Autodesk Inventor part; units mm, degrees
ref_plane "YZ Plane" through (0, 0, 0) normal (1, 0, 0) x (0, 1, 0)
ref_plane "XZ Plane" through (0, 0, 0) normal (0, 1, 0) x (-1, 0, 0)
ref_plane "XY Plane" through (0, 0, 0) normal (0, 0, 1) x (1, 0, 0)
sketch "Szkic1" plane through (0, 0, 0) normal (0, 0, 1) x (1, 0, 0)
  circle A0 centre (0, 0) radius 30
  circle A1 centre (0, 0) radius 34
  dimension "d0" = 60
  dimension "d1" = 4
extrude "Wyciągnięcie proste1" add sketch "Szkic1" along normal blind 65
sketch "Szkic2" plane through (0, 0, 65) normal (0, 0, 1) x (1, 0, 0)
  circle A0 centre (35, 0) radius 5
  circle A1 centre (0, 0) radius 34
  circle A2 centre (0, 0) radius 30
  circle A3 centre (35, 0) radius 1.5
  line L0 (0, 0) -> (0, -30)
  circle A4 centre (-35, 0) radius 5
  circle A5 centre (-35, 0) radius 1.5
  point P0 (33.9821, 1.1018)
  point P1 (33.9821, -1.1018)
  point P2 (33.6571, -4.8163)
  point P3 (33.6571, 4.8163)
  point P4 (-33.9821, -1.1018)
  point P5 (-33.9821, 1.1018)
  point P6 (-33.6571, 4.8163)
  point P7 (-33.6571, -4.8163)
  dimension "d5" = 10
  dimension "d6" = 3
  dimension "d9" = 70
extrude "Wyciągnięcie proste2" add sketch "Szkic2" against normal blind 10 contours A0 A1 A3 | A1 A5 A4 picked at (35.0063, -3.323) picked at (-35.0802, 3.3077)
sketch "Szkic3" plane through (0, 0, 65) normal (0, 0, 1) x (1, 0, 0)
  point P0 (0, 0)
sketch "Szkic4" plane through (0, 0, 65) normal (0, 0, 1) x (1, 0, 0)
  arc A0 (-33.9821, 1.1018) -> (-33.9821, -1.1018) centre (-35, 0) ccw
  circle A1 centre (-35, 0) radius 1.5
  arc A2 (33.9821, -1.1018) -> (33.9821, 1.1018) centre (35, 0) ccw
  circle A3 centre (35, 0) radius 1.5
  point P0 (0, 0)
  point P1 (33.9821, 1.1018)
  point P2 (33.9821, -1.1018)
  point P3 (-33.9821, -1.1018)
  point P4 (-33.9821, 1.1018)
extrude "Wyciągnięcie proste3" cut sketch "Szkic4" against normal blind 10
properties part number "osłonasilnik" material "Tworzywo sztuczne PET"
Can you work these out from the model? Positions are in its coordinate system, mm. A direction names the side the tool comes from. Coordinates: 2 decimals unless noted, no trailing zeros. Write each loop counter-clockwise with the first axis right and the second up, starting at its lowest first coordinate (ties: lowest second). Pieces come first, ordered by that corner, then holes. Notation, with made-up numbers: (-27.75, -17) - (30.25, -17) arc R21 cw to (30.25, 19) - close; hole circle Ø1 at (23.25, 26.5). An arc over 180 degrees is marked (long way). Return JSON: item names as keys, results as strings. Group by question number.
Item 1: If we section it at D-D (z = 56): Write out the boundary of the cut face in (x, y).
Item 2: I'm going to push flat-ended pins straight in: pin 1 Ø1.5 at (y, z) = (12.5, 7) entering from +X; pin 2 Ø5 at (x, z) = (29.5, 25) entering from -Y; pin 3 Ø8 at (x, z) = (22, 16.5) entering from -Y. Where does each tip first touch, or does it pass through?
Item 3: We'd pull the mould along Y, two halves only. Please class faces 3 (the face through (32.43, -10.21, 32.04)), 4 (the face through (-37, 0, 55)), 5 (the face through (36.5, 0, 60.1)): pulls with the +Y half, pulls with the -Y half, needs draft (parallel to the pull), parting line crosses it, or undercut.
Item 4: Please list where these lines run through material, in increasing order: probe 1 along Y at (x, z) = (0, 39.5); probe 2 along X at (y, z) = (1, 30.5); probe 3 along Y at (x, z) = (-35, 63).
Item 5: If we section it at B-B (y = 0): Write out the boundary of the cut face in (x, z), then the cut area to 3 significant figures.
Item 6: Which directions (+Z, -Z, +X, -X, +Y, -Y) give clear straight access to the entire face, cutting with the end or side of a thin tool? Please do faces 1 (the face through (-29.97, -1.32, 32.04)), 2 (the face through (33.8, 0, 55)).
Item 7: If we section it at C-C (y = -25): Write out the boundary of the cut face in (x, z), then the cut area to 3 significant figures.
Item 8: If we section it at A-A (x = 0): Write out the boundary of the cut face in (y, z), then the cut area to 3 significant figures.
Return value:
{
 "1": {"outline": "(-33.66, -4.82) arc R34 ccw to (33.66, -4.82) arc R5 ccw (long way) to (33.66, 4.82) arc R34 ccw to (-33.66, 4.82) arc R5 ccw (long way) to start; hole circle Ø3 at (-35, 0); hole circle Ø60 at (0, 0); hole circle Ø3 at (35, 0)"},
 "2": {"pin 1": "stops at x = 31.91", "pin 2": "stops at y = -20.66", "pin 3": "stops at y = -28.84"},
 "3": {"face 3": "parting line crosses it", "face 4": "needs draft", "face 5": "undercut"},
 "4": {"probe 1": "y = -34 to -30, 30 to 34", "probe 2": "x = -33.99 to -29.98, 29.98 to 33.99", "probe 3": "y = -5 to -1.5, 1.5 to 5"},
 "5": {"outline": "(-40, 55) - (-36.5, 55) - (-36.5, 65) - (-40, 65) - close; (-34, 0) - (-30, 0) - (-30, 65) - (-33.5, 65) - (-33.5, 55) - (-34, 55) - close; (30, 0) - (34, 0) - (34, 55) - (33.5, 55) - (33.5, 65) - (30, 65) - close; (36.5, 55) - (40, 55) - (40, 65) - (36.5, 65) - close", "area": "580 mm^2"},
 "6": {"face 1": "+Z, -Z", "face 2": "+Z"},
 "7": {"outline": "(-23.04, 0) - (-16.58, 0) - (-16.58, 65) - (-23.04, 65) - close; (16.58, 0) - (23.04, 0) - (23.04, 65) - (16.58, 65) - close", "area": "840 mm^2"},
 "8": {"outline": "(-34, 0) - (-30, 0) - (-30, 65) - (-34, 65) - close; (30, 0) - (34, 0) - (34, 65) - (30, 65) - close", "area": "520 mm^2"}
}
